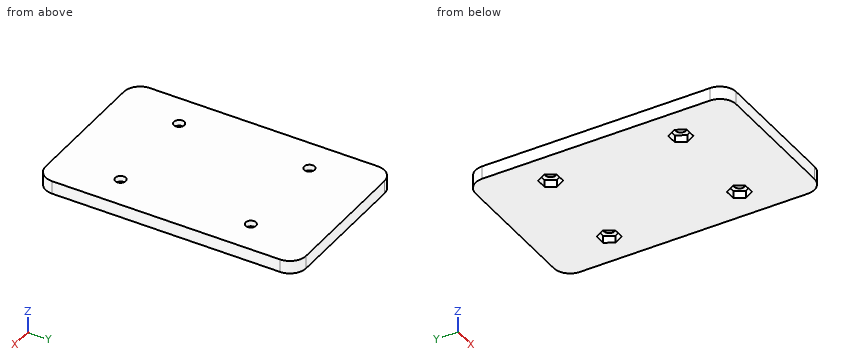
```python
from build123d import *

# Parameters (mm, degrees)
DODANIE_WYCI_GNI_CIE1_DEPTH = 4
WYTNIJ_WYCI_GNI_CIE1_REACH  = 49.339
SZKIC2_R                    = 1.6
SZKIC3_R                    = 1.6
WYTNIJ_WYCI_GNI_CIE2_DEPTH  = 2.2


with BuildPart() as part:
    # Szkic1 → Dodanie-wyciągnięcie1 (new body)
    with BuildSketch(Plane.XY):
        with BuildLine():
            Line((-20, -40), (20, -40))
            ThreePointArc((20, -40), (23.535533906, -38.535533906), (25, -35))
            Line((25, -35), (25, 35))
            ThreePointArc((25, 35), (23.535533906, 38.535533906), (20, 40))
            Line((20, 40), (-20, 40))
            ThreePointArc((-20, 40), (-23.535533906, 38.535533906), (-25, 35))
            Line((-25, 35), (-25, -35))
            ThreePointArc((-25, -35), (-23.535533906, -38.535533906), (-20, -40))
        make_face()
    extrude(amount=DODANIE_WYCI_GNI_CIE1_DEPTH)

    # Szkic2 → Wytnij-wyciągnięcie1 (cut, up to next)
    with BuildSketch(Plane(origin=(0, 0, 0), x_dir=(-1, 0, 0), z_dir=(0, 0, -1)), mode=Mode.PRIVATE) as wytnij_wyci_gni_cie1_sk1:
        with Locations((-15, 20)):
            Circle(SZKIC2_R)
    wytnij_wyci_gni_cie1_tool1 = extrude(wytnij_wyci_gni_cie1_sk1.sketch, amount=-WYTNIJ_WYCI_GNI_CIE1_REACH, mode=Mode.PRIVATE) & part.part
    # Szkic2 → Wytnij-wyciągnięcie1 (cut, up to next)
    with BuildSketch(Plane(origin=(0, 0, 0), x_dir=(-1, 0, 0), z_dir=(0, 0, -1)), mode=Mode.PRIVATE) as wytnij_wyci_gni_cie1_sk2:
        with Locations(Location((15, 20, 0), (0, 0, 180))):
            Circle(SZKIC2_R)
    wytnij_wyci_gni_cie1_tool2 = extrude(wytnij_wyci_gni_cie1_sk2.sketch, amount=-WYTNIJ_WYCI_GNI_CIE1_REACH, mode=Mode.PRIVATE) & part.part
    # Szkic2 → Wytnij-wyciągnięcie1 (cut, up to next)
    with BuildSketch(Plane(origin=(0, 0, 0), x_dir=(-1, 0, 0), z_dir=(0, 0, -1)), mode=Mode.PRIVATE) as wytnij_wyci_gni_cie1_sk3:
        with Locations((15, -20)):
            Circle(SZKIC2_R)
    wytnij_wyci_gni_cie1_tool3 = extrude(wytnij_wyci_gni_cie1_sk3.sketch, amount=-WYTNIJ_WYCI_GNI_CIE1_REACH, mode=Mode.PRIVATE) & part.part
    # Szkic2 → Wytnij-wyciągnięcie1 (cut, up to next)
    with BuildSketch(Plane(origin=(0, 0, 0), x_dir=(-1, 0, 0), z_dir=(0, 0, -1)), mode=Mode.PRIVATE) as wytnij_wyci_gni_cie1_sk4:
        with Locations(Location((-15, -20, 0), (0, 0, 180))):
            Circle(SZKIC2_R)
    wytnij_wyci_gni_cie1_tool4 = extrude(wytnij_wyci_gni_cie1_sk4.sketch, amount=-WYTNIJ_WYCI_GNI_CIE1_REACH, mode=Mode.PRIVATE) & part.part
    add(wytnij_wyci_gni_cie1_tool1.solids().sort_by_distance((15, 20, 0))[0], mode=Mode.SUBTRACT)
    add(wytnij_wyci_gni_cie1_tool2.solids().sort_by_distance((-15, 20, 0))[0], mode=Mode.SUBTRACT)
    add(wytnij_wyci_gni_cie1_tool3.solids().sort_by_distance((-15, -20, 0))[0], mode=Mode.SUBTRACT)
    add(wytnij_wyci_gni_cie1_tool4.solids().sort_by_distance((15, -20, 0))[0], mode=Mode.SUBTRACT)

    # Szkic3 → Wytnij-wyciągnięcie2 (cut)
    # profile 1 of 4: a face of its own
    with BuildSketch(Plane(origin=(0, 0, 0), x_dir=(-1, 0, 0), z_dir=(0, 0, -1))):
        Polygon((-11.709103466, 20), (-13.354551733, 22.85), (-16.645448267, 22.85), (-18.290896534, 20), (-16.645448267, 17.15), (-13.354551733, 17.15), align=None)
        with Locations((-15, 20)):
            Circle(SZKIC3_R, mode=Mode.SUBTRACT)
    # profile 2 of 4: a face of its own
    with BuildSketch(Plane(origin=(0, 0, 0), x_dir=(-1, 0, 0), z_dir=(0, 0, -1))):
        Polygon((13.354551733, 17.15), (11.709103466, 20), (13.354551733, 22.85), (16.645448267, 22.85), (18.290896534, 20), (16.645448267, 17.15), align=None)
        with Locations(Location((15, 20, 0), (0, 0, 180))):
            Circle(SZKIC3_R, mode=Mode.SUBTRACT)
    # profile 3 of 4: a face of its own
    with BuildSketch(Plane(origin=(0, 0, 0), x_dir=(-1, 0, 0), z_dir=(0, 0, -1))):
        Polygon((11.709103466, -20), (13.354551733, -22.85), (16.645448267, -22.85), (18.290896534, -20), (16.645448267, -17.15), (13.354551733, -17.15), align=None)
        with Locations((15, -20)):
            Circle(SZKIC3_R, mode=Mode.SUBTRACT)
    # profile 4 of 4: a face of its own
    with BuildSketch(Plane(origin=(0, 0, 0), x_dir=(-1, 0, 0), z_dir=(0, 0, -1))):
        Polygon((-13.354551733, -17.15), (-11.709103466, -20), (-13.354551733, -22.85), (-16.645448267, -22.85), (-18.290896534, -20), (-16.645448267, -17.15), align=None)
        with Locations(Location((-15, -20, 0), (0, 0, 180))):
            Circle(SZKIC3_R, mode=Mode.SUBTRACT)
    extrude(amount=-WYTNIJ_WYCI_GNI_CIE2_DEPTH, mode=Mode.SUBTRACT)


solid = part.part
```
Read the model definition and answer for the solid it produces. Units are mm, in the model's axes. Coordinates: 2 decimals unless noted, no trailing zeros. Write each loop counter-clockwise with the first axis right and the second up, starting at its lowest first coordinate (ties: lowest second). Pieces come first, ordered by that corner, then holes. Notation, with made-up numbers: (36.25, 36.25) - (52.25, 36.25) arc R30 ccw to (52.25, 66.25) - close; hole circle Ø7 at (18, 20). An arc over 180 degrees is marked (long way). Answer as a JSON object with one key per item and string values. Group by question number.
1. A cutting plane is placed at A-A (x = 15). Determine the outline of the cut face in (y, z), plus the area to 3 significant figures.
2. This flat-tipped pin is pushed along its axis until it touches: P1, Ø4, axis at x = 15, y = 20, coming from the -Z side. Where does it stop, or does it pass through?
3. Consider L1, parallel to Y at x = 15, z = 2.7; L2, parallel to Z at x = 13, y = 20; L3, parallel to Y at x = -20.5, z = 0.5. Determine where each line is inside the solid, lowest interval first. Write a range as [from, to].
Worked out:
{
 "1": {"outline": "(-40, 0) - (-22.85, 0) - (-22.85, 2.2) - (-21.6, 2.2) - (-21.6, 4) - (-40, 4) - close; (-18.4, 2.2) - (-17.15, 2.2) - (-17.15, 0) - (17.15, 0) - (17.15, 2.2) - (18.4, 2.2) - (18.4, 4) - (-18.4, 4) - close; (21.6, 2.2) - (22.85, 2.2) - (22.85, 0) - (40, 0) - (40, 4) - (21.6, 4) - close", "area": "283 mm²"},
 "2": {"P1": "stops at z = 2.2"},
 "3": {"L1": "y = [-40, -21.6], [-18.4, 18.4], [21.6, 40]", "L2": "z = [2.2, 4]", "L3": "y = [-39.97, 39.97]"}
}
